Verification items for the finished model (mm, model axes). Give positions to 0.01 mm unless a question says otherwise; leave off trailing zeros. Write item = value, one per line.
from build123d import *

# Parameters (mm, degrees)
F0_R     = 11
F1_DEPTH = 7
F2_R     = 12.499
F3_SIZE  = 2


# Not quite as in the source:
# - a fillet or chamfer is up to 0.001 mm smaller than in the source, because OpenCascade refuses the exact size


with BuildPart() as f1:
    # F0 (on Top) → F1 (new body)
    with BuildSketch(Plane.XY):
        with BuildLine():
            ThreePointArc((14.9052440041, -1.6833600857), (14.9762922658, -0.8430124372), (15, 0))
            ThreePointArc((15, 0), (12.5483433381, 8.2182163192), (5.9947894041, 13.75))
            ThreePointArc((5.9947894041, 13.75), (0, 12.5), (-5.9947894041, 13.75))
            ThreePointArc((-5.9947894041, 13.75), (-12.9903810568, 7.5), (-14.9052440041, -1.6833600857))
            ThreePointArc((-14.9052440041, -1.6833600857), (-10.8253175473, -6.25), (-8.9104546, -12.0666399143))
            ThreePointArc((-8.9104546, -12.0666399143), (0, -15), (8.9104546, -12.0666399143))
            ThreePointArc((8.9104546, -12.0666399143), (10.8253175473, -6.25), (14.9052440041, -1.6833600857))
        make_face()
        Circle(F0_R, mode=Mode.SUBTRACT)
        with BuildLine():
            ThreePointArc((-5.9947894041, 13.75), (0, 12.5), (5.9947894041, 13.75))
            ThreePointArc((5.9947894041, 13.75), (0, 15), (-5.9947894041, 13.75))
        make_face()
        with BuildLine():
            ThreePointArc((-5.9947894041, 13.75), (0, 15), (5.9947894041, 13.75))
            ThreePointArc((5.9947894041, 13.75), (12.5483433381, 19.2817836808), (15, 27.5))
            ThreePointArc((15, 27.5), (-8.2182163192, 40.0483433381), (-5.9947894041, 13.75))
        make_face()
        with BuildLine():
            ThreePointArc((38.8156986041, -13.75), (30.5737745507, -0.3586442247), (14.9052440041, -1.6833600857))
            ThreePointArc((14.9052440041, -1.6833600857), (12.9903810568, -7.5), (8.9104546, -12.0666399143))
            ThreePointArc((8.9104546, -12.0666399143), (22.9726861669, -28.7262922658), (38.8156986041, -13.75))
        make_face()
        with BuildLine():
            ThreePointArc((8.9104546, -12.0666399143), (12.9903810568, -7.5), (14.9052440041, -1.6833600857))
            ThreePointArc((14.9052440041, -1.6833600857), (10.8253175473, -6.25), (8.9104546, -12.0666399143))
        make_face()
        with BuildLine():
            ThreePointArc((-8.9104546, -12.0666399143), (-10.8253175473, -6.25), (-14.9052440041, -1.6833600857))
            ThreePointArc((-14.9052440041, -1.6833600857), (-12.9903810568, -7.5), (-8.9104546, -12.0666399143))
        make_face()
        with BuildLine():
            ThreePointArc((-8.9104546, -12.0666399143), (-12.9903810568, -7.5), (-14.9052440041, -1.6833600857))
            ThreePointArc((-14.9052440041, -1.6833600857), (-37.2070543793, -20.5080759466), (-8.8156986041, -13.75))
            ThreePointArc((-8.8156986041, -13.75), (-8.8394063383, -12.9069875628), (-8.9104546, -12.0666399143))
        make_face()
    extrude(amount=F1_DEPTH)

    # F2 (radius 12.5 in the source; OpenCascade refuses exactly that, so slightly less here)
    f2_edges = [f1.edges().sort_by_distance(p)[0] for p in [
        (-5.994789, 13.75, 3.5),
        (14.905244, -1.68336, 3.5),
        (-14.905244, -1.68336, 3.5),
        (5.994789, 13.75, 3.5),
        (-8.910455, -12.06664, 3.5),
        (8.910455, -12.06664, 3.5),
    ]]
    fillet(f2_edges, radius=F2_R)

    # F3
    f3_edges = [f1.edges().sort_by_distance(p)[0] for p in [
        (-6.250077, -16.674548, 0),
        (-6.250077, -16.674548, 7),
    ]]
    chamfer(f3_edges, length=F3_SIZE)


solid = f1.part
1) Draft check along X on faces 1 (the cylindrical face through (-37, -20.9, 3.5)), 2 (the conical face through (-35.37, -19.976, 6.875)), 3 (the flat face through (-9, -8, 7)). Enter one of: +X half, -X half, draft (parallel to the pull), parting line (faces both ways), or undercut.
From the geometry:
face_1 = undercut
face_2 = undercut
face_3 = draft
2) Material ranges on probe 1 along Y at (x, z) = (0, 2.25); probe 2 along Y at (x, z) = (8, 5.75); probe 3 along X at (y, z) = (7, 1.25), recorded low to high. Write a range as from..to.
From the geometry:
probe_1 = -15..-11, 11..42.5
probe_2 = -16.94..-7.55, 7.55..39.29
probe_3 = -12.41..-8.49, 8.49..12.41
3) Depth check by flat-ended pin: P1, Ø3, axis at y = 15, z = 2, coming from the +X side; P2, Ø1.5, axis at y = -15, z = 1, coming from the -X side; P3, Ø3, axis at y = 30, z = 1, coming from the +X side. Enter the tip coordinate at first touch or a pass-through.
From the geometry:
P1 = 11.62
P2 = -38.52
P3 = 14.94
